from build123d import *

# Parameters (mm, degrees)
SKETCH1_R           = 36
SKETCH1_R_2         = 20.52
BOSS_EXTRUDE1_DEPTH = 20
SKETCH2_W           = 2056.908092605
SKETCH2_H           = 385.28
BOSS_EXTRUDE2_DEPTH = 10
BOSS_EXTRUDE3_START = 30
SKETCH3_R           = 36
BOSS_EXTRUDE3_DEPTH = 30
SKETCH4_W           = 2013.042913478
SKETCH4_H           = 345.28
BOSS_EXTRUDE4_DEPTH = 10


with BuildPart() as part:
    # Sketch1 → Boss-Extrude1 (new body)
    with BuildSketch(Plane.XY):
        Polygon((-406.4, -152.64), (406.4, -152.64), (1650.508092605, -152.64), (1650.508092605, 232.64), (-406.4, 232.64), (-406.4, 152.64), align=None)
        Circle(SKETCH1_R, mode=Mode.SUBTRACT)
        with Locations((0, 95.04)):
            Circle(SKETCH1_R_2, mode=Mode.SUBTRACT)
        with Locations((0, -95.04)):
            Circle(SKETCH1_R_2, mode=Mode.SUBTRACT)
    extrude(amount=BOSS_EXTRUDE1_DEPTH)

    # Sketch2 → Boss-Extrude2 (add)
    with BuildSketch(Plane.XY.offset(20)):
        with Locations((622.054046302, 40)):
            Rectangle(SKETCH2_W, SKETCH2_H)
    extrude(amount=BOSS_EXTRUDE2_DEPTH)

    # Sketch3 → Boss-Extrude3 (add)
    with BuildSketch(Plane(origin=(0, 0, 20), x_dir=(-1, 0, 0), z_dir=(0, 0, -1)).offset(BOSS_EXTRUDE3_START)):
        with Locations(Location((0, 0, 0), (0, 0, 180))):
            Circle(SKETCH3_R)
    extrude(amount=-BOSS_EXTRUDE3_DEPTH)

    # Sketch4 → Boss-Extrude4 (add)
    with BuildSketch(Plane(origin=(0, 0, 0), x_dir=(-1, 0, 0), z_dir=(0, 0, -1))):
        Polygon((-1630.508092605, 232.64), (-1650.508092605, 232.64), (-1650.508092605, -152.64), (403.233696812, -152.64), (403.233696812, 232.64), align=None)
        with Locations((-623.986635866, 40)):
            Rectangle(SKETCH4_W, SKETCH4_H, mode=Mode.SUBTRACT)
    extrude(amount=BOSS_EXTRUDE4_DEPTH)


solid = part.part
Verification items for the finished model (mm, model axes). A direction names the side the tool comes from. Round coordinates to 2 decimals unless told otherwise and drop trailing zeros. Order: outer loops, then holes, each group sorted by start corner. A loop starts at its lowest first (then second) coordinate and runs counter-clockwise, first axis right, second up.
1. Thickness scan on L1, parallel to Y at x = 0, z = 6; L2, parallel to X at y = 95, z = 9; L3, parallel to Y at x = -223, z = -1. Record the ranges inside material, lowest first.
Final values:
L1: y = -152.64 to -115.56, -74.52 to 74.52, 115.56 to 232.64
L2: x = -406.4 to -20.52, 20.52 to 1650.51
L3: y = -152.64 to -132.64, 212.64 to 232.64
2. Section check B-B on y = -95.04. Record the cut outline in (x, z), then the cut area to 3 significant figures.
Final values:
outline: (-406.4, 0) - (-403.23, 0) - (-403.23, -10) - (-382.53, -10) - (-382.53, 0) - (-20.52, 0) - (-20.52, 20) - (20.52, 20) - (20.52, 0) - (1630.51, 0) - (1630.51, -10) - (1650.51, -10) - (1650.51, 30) - (-406.4, 30) - close
area: 61,300 mm2
3. Release check for a two-part mould opening along Y. For faces 3 (the flat face through (1650.508, 43, 10)), 4 (the flat face through (608, 232.64, 10)), 5 (the flat face through (0, -95, 20)) record: +Y half, -Y half, draft (parallel to the pull), parting line (faces both ways), or undercut.
Final values:
face 3: draft
face 4: +Y half
face 5: undercut
4. Go/stop test with flat-tipped pins: P1, Ø0.9, axis at x = -405.5, y = -51.5, coming from the -Z side; P2, Ø24.5, axis at x = 0, y = 95.04, coming from the -Z side; P3, Ø3, axis at y = 105, z = -5.5, coming from the -X side. Record where each tip stops, or that it passes through.
Final values:
P1: stops at z = 0
P2: stops at z = 20
P3: stops at x = -403.23
5. Access from +Z, -Z, +X, -X, +Y, -Y to the whole of each face (thin tool, end or side, straight path). Record for faces 1 (the flat face through (610, 42, 0)), 2 (the flat face through (-1, -1, -10)).
Final values:
face 1: -Z
face 2: -Z, +X, -X, +Y, -Y
6. Section check A-A on x = 0. Record the cut outline in (y, z), then the cut area to 3 significant figures.
Final values:
outline: (-152.64, -10) - (-132.64, -10) - (-132.64, 0) - (-115.56, 0) - (-115.56, 20) - (-74.52, 20) - (-74.52, 0) - (-36, 0) - (-36, -10) - (36, -10) - (36, 0) - (74.52, 0) - (74.52, 20) - (115.56, 20) - (115.56, 0) - (212.64, 0) - (212.64, -10) - (232.64, -10) - (232.64, 30) - (-152.64, 30) - close
area: 11,000 mm2
7. Section check C-C on x = 1227. Record the cut outline in (y, z).
Final values:
outline: (-152.64, -10) - (-132.64, -10) - (-132.64, 0) - (212.64, 0) - (212.64, -10) - (232.64, -10) - (232.64, 30) - (-152.64, 30) - close
